Can you work these out from the model? Positions are in its coordinate system, mm. A direction names the side the tool comes from. Round coordinates to 2 decimals unless told otherwise and drop trailing zeros. Order: outer loops, then holes, each group sorted by start corner. A loop starts at its lowest first (then second) coordinate and runs counter-clockwise, first axis right, second up. Notation, with made-up numbers: (64, -22.75) -> (79, -22.75) arc R21 cw to (79, -4.75) -> close; hole circle Ø4 at (76.25, 7). An arc over 180 degrees is marked (long way). One line per item, written item: value.
```python
from build123d import *

# Parameters (mm, degrees)
SKETCH1_R           = 2
BOSS_EXTRUDE1_DEPTH = 2
SKETCH2_R           = 2.391473365
SKETCH2_R_2         = 2
SKETCH2_R_3         = 0.308853545
BOSS_EXTRUDE2_DEPTH = 1
FILLET1_R           = 0.2
SKETCH3_R           = 0.25
BOSS_EXTRUDE3_DEPTH = 2


with BuildPart() as part:
    # Sketch1 → Boss-Extrude1 (new body)
    with BuildSketch(Plane.XY):
        Polygon((0, -7.1), (5.1, -7.1), (5.1, 0), (5.1, 2.55), (2.55, 5.1), (-2.55, 5.1), (-5.1, 2.55), (-5.1, 0), (-5.1, -7.1), align=None)
        Circle(SKETCH1_R, mode=Mode.SUBTRACT)
    extrude(amount=BOSS_EXTRUDE1_DEPTH)

    # Sketch2 → Boss-Extrude2 (add)
    # profile 1 of 3: a face of its own
    with BuildSketch(Plane.XY.offset(2)):
        Circle(SKETCH2_R)
        Circle(SKETCH2_R_2, mode=Mode.SUBTRACT)
    # profile 2 of 3: a face of its own
    with BuildSketch(Plane.XY.offset(2)):
        with Locations((-4.567781371, -6.437447931)):
            Circle(SKETCH2_R_3)
    # profile 3 of 3: a face of its own
    with BuildSketch(Plane.XY.offset(2)):
        with Locations(Location((4.567781371, -6.437447931, 0), (0, 0, 180))):
            Circle(SKETCH2_R_3)
    extrude(amount=BOSS_EXTRUDE2_DEPTH)

    # Fillet1
    fillet1_edges = [part.edges().sort_by_distance(p)[0] for p in [
        (-4.876634915, -6.437447931, 2),
        (4.876634915, -6.437447931, 2),
        (-2.391473365, 0, 2),
    ]]
    fillet(fillet1_edges, radius=FILLET1_R)

    # Sketch3 → Boss-Extrude3 (add)
    with BuildSketch(Plane.XZ.offset(7.1)):
        with Locations(Location((0, 1.75, 0), (0, 0, 90))):
            Circle(SKETCH3_R)
        with Locations(Location((2, 1.75, 0), (0, 0, 90))):
            Circle(SKETCH3_R)
        with Locations(Location((-2, 1.75, 0), (0, 0, 180))):
            Circle(SKETCH3_R)
    extrude(amount=BOSS_EXTRUDE3_DEPTH)


solid = part.part
```
Q1. On a 3-axis mill with a long thin cutter (end or side, diameter ignored), from which of +Z, -Z, +X, -X, +Y, -Y can I reach the whole of each face in a straight line? I mean faces 1 (the face through (0, -4, 2)), 2 (the face through (-3.81, 3.84, 0.99)). Say none if no direction works.
Answers below:
face 1: +Z
face 2: +Z, -Z, -X, +Y
Q2. Please list where these lines run through material, in increasing order: line 1 along Y through (x, z) = (0, 1.65); line 2 along Y through (x, z) = (0, 1.25); line 3 along Z through (x, y) = (-1.5, -4.75).
Answers below:
line 1: -9.1 to -2, 2 to 5.1
line 2: -7.1 to -2, 2 to 5.1
line 3: 0 to 2
Q3. I want a section at C-C on z = 0.6. List the corners of the cut face in (x, y) for me, plus the area to 3 significant figures.
Answers below:
outline: (-5.1, -7.1) -> (5.1, -7.1) -> (5.1, 2.55) -> (2.55, 5.1) -> (-2.55, 5.1) -> (-5.1, 2.55) -> close; hole circle Ø4 at (0, 0)
area: 105 mm^2
Q4. We'd pull the mould along X, two halves only. Please class faces 3 (the face through (-5.1, -2, 1)), 4 (the face through (-1, -2, 3)), 5 (the face through (-0.518, -2.335, 2.594)), 6 (the face through (0, -2, 1)): released by +X, released by -X, zero draft, split by the parting line, or undercut.
Answers below:
face 3: released by -X
face 4: zero draft
face 5: split by the parting line
face 6: undercut
Q5. I want a section at B-B on y = -8. List the corners of the cut face in (x, z) for me.
Answers below:
outline: circle Ø0.5 at (-2, 1.75); circle Ø0.5 at (0, 1.75); circle Ø0.5 at (2, 1.75)
Q6. I want a section at A-A on z = 1.75. List the corners of the cut face in (x, y) for me.
Answers below:
outline: (-5.1, -7.1) -> (-2.25, -7.1) -> (-2.25, -9.1) -> (-1.75, -9.1) -> (-1.75, -7.1) -> (-0.25, -7.1) -> (-0.25, -9.1) -> (0.25, -9.1) -> (0.25, -7.1) -> (1.75, -7.1) -> (1.75, -9.1) -> (2.25, -9.1) -> (2.25, -7.1) -> (5.1, -7.1) -> (5.1, 2.55) -> (2.55, 5.1) -> (-2.55, 5.1) -> (-5.1, 2.55) -> close; hole circle Ø4 at (0, 0)
Q7. I want a section at D-D on y = 3. List the corners of the cut face in (x, z) for me.
Answers below:
outline: (-4.65, 0) -> (4.65, 0) -> (4.65, 2) -> (-4.65, 2) -> close
